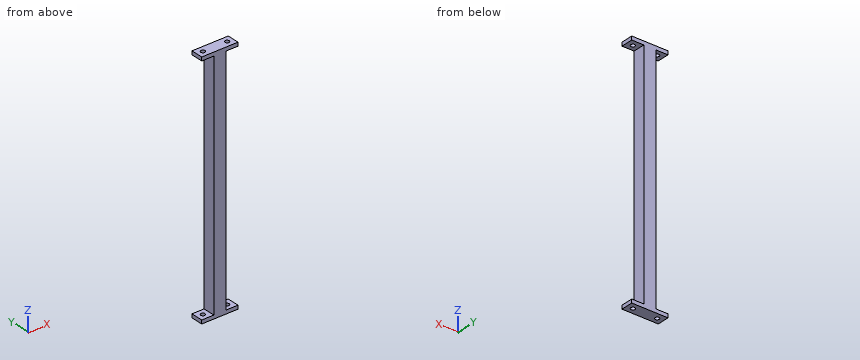
```python
from build123d import *

# Parameters (mm, degrees)
SKETCH_1_W          = 10
SKETCH_1_H          = 10
SKETCH_1_R          = 1.75
EXTRUDE_1_DEPTH     = 200
SKETCH_2_W          = 194
SKETCH_2_H          = 10
CUT_EXTRUDE_1_DEPTH = 10
SKETCH_3_W          = 194
SKETCH_3_H          = 10
CUT_EXTRUDE_2_DEPTH = 10


with BuildPart() as part:
    # 草图1 → 凸台-拉伸1 (new body)
    # profile 1 of 3: a face of its own
    with BuildSketch(Plane.XY):
        Rectangle(SKETCH_1_W, SKETCH_1_H)
    # profile 2 of 3: a face of its own
    with BuildSketch(Plane.XY):
        with Locations((-10, 0)):
            Rectangle(SKETCH_1_W, SKETCH_1_H)
        with Locations(Location((-10, 0, 0), (0, 0, 180))):
            Circle(SKETCH_1_R, mode=Mode.SUBTRACT)
    # profile 3 of 3: a face of its own
    with BuildSketch(Plane.XY):
        with Locations((10, 0)):
            Rectangle(SKETCH_1_W, SKETCH_1_H)
        with Locations((10, 0)):
            Circle(SKETCH_1_R, mode=Mode.SUBTRACT)
    extrude(amount=EXTRUDE_1_DEPTH)

    # 草图2 → 切除-拉伸1 (cut)
    with BuildSketch(Plane(origin=(15, 0, 0), x_dir=(0, 0, -1), z_dir=(1, 0, 0))):
        with Locations((-100, 0)):
            Rectangle(SKETCH_2_W, SKETCH_2_H)
    extrude(amount=-CUT_EXTRUDE_1_DEPTH, mode=Mode.SUBTRACT)

    # 草图3 → 切除-拉伸2 (cut)
    with BuildSketch(Plane.ZY.offset(15)):
        with Locations((100, 0)):
            Rectangle(SKETCH_3_W, SKETCH_3_H)
    extrude(amount=-CUT_EXTRUDE_2_DEPTH, mode=Mode.SUBTRACT)


solid = part.part
```
Could you check a few things on this model? Use its own coordinates, in mm. Coordinates: 2 decimals unless noted, no trailing zeros. Loops run counter-clockwise (first coordinate to the right, second up) from the corner with the lowest first, then second, coordinate; pieces in that order, holes last.
1) Imagine slicing it at C-C (z = 18). List the corners of the cut face in (x, y) for me.
Reported:
outline: (-5, -5) - (5, -5) - (5, 5) - (-5, 5) - close
2) Will these pins go through, and if not, where does the flat tip stop? pin 1 Ø3 at (x, y) = (-12, 0) entering from -Z; pin 2 Ø1 at (y, z) = (2, 86.5) entering from +X; pin 3 Ø2 at (y, z) = (0, 171.5) entering from -X; pin 4 Ø3 at (x, y) = (10, 0) entering from +Z.
Reported:
pin 1: stops at z = 0
pin 2: stops at x = 5
pin 3: stops at x = -5
pin 4: passes through
3) Imagine slicing it at B-B (y = 0). List the corners of the cut face in (x, z) for me, and give its area (3 significant figures).
Reported:
outline: (-15, 0) - (-11.75, 0) - (-11.75, 3) - (-15, 3) - close; (-15, 197) - (-11.75, 197) - (-11.75, 200) - (-15, 200) - close; (-8.25, 0) - (8.25, 0) - (8.25, 3) - (5, 3) - (5, 197) - (8.25, 197) - (8.25, 200) - (-8.25, 200) - (-8.25, 197) - (-5, 197) - (-5, 3) - (-8.25, 3) - close; (11.75, 0) - (15, 0) - (15, 3) - (11.75, 3) - close; (11.75, 197) - (15, 197) - (15, 200) - (11.75, 200) - close
area: 2,080 mm2
4) Imagine slicing it at A-A (x = -10). List the corners of the cut face in (y, z) for me, and give its area (3 significant figures).
Reported:
outline: (-5, 0) - (-1.75, 0) - (-1.75, 3) - (-5, 3) - close; (-5, 197) - (-1.75, 197) - (-1.75, 200) - (-5, 200) - close; (1.75, 0) - (5, 0) - (5, 3) - (1.75, 3) - close; (1.75, 197) - (5, 197) - (5, 200) - (1.75, 200) - close
area: 39.0 mm2
5) Please list where these lines run through material, in increasing order: line 1 along Y through (x, z) = (10, 198.9); line 2 along Z through (x, y) = (13.75, -3.75); line 3 along X through (y, z) = (-4, 186.5).
Reported:
line 1: y = -5 to -1.75, 1.75 to 5
line 2: z = 0 to 3, 197 to 200
line 3: x = -5 to 5
